Check sheet for the modelled part. Datum: model origin and axes. Units: mm. Face numbers are marked on the shaded views. A direction names the side the tool comes from. Round coordinates to 2 decimals unless told otherwise and drop trailing zeros. Write each loop counter-clockwise with the first axis right and the second up, starting at its lowest first coordinate (ties: lowest second). Pieces come first, ordered by that corner, then holes. Notation, with made-up numbers: M 29,16 L 49,16 A20 cw 49,33 Z; hole C 58.25,42 d3. An arc over 180 degrees is marked long. Answer in a Markdown table with one row per item.
```python
from build123d import *

# Parameters (mm, degrees)
F0_W     = 60
F0_H     = 30
F1_DEPTH = 30
F2_T     = -1.5
F3_R     = 6
F4_DEPTH = 1.501
F5_R     = 4
F6_DEPTH = 30.001
F7_R     = 2
F8_SIZE  = 1


with BuildPart() as f1:
    # F0 (on Top) → F1 (new body)
    with BuildSketch(Plane.XY):
        Rectangle(F0_W, F0_H)
    extrude(amount=F1_DEPTH)

    # F2
    f2_openings = [f1.faces().sort_by_distance(p)[0] for p in [
        (0, 0, 0),
    ]]
    offset(amount=F2_T, openings=f2_openings)

    # F3 (on face) → F4 (cut, through all)
    with BuildSketch(Plane(origin=(0, -13.5, 0), x_dir=(-1, 0, 0), z_dir=(0, 1, 0))):
        with Locations((-18.5, 19.5)):
            Circle(F3_R)
        with Locations((18.5, 19.5)):
            Circle(F3_R)
    extrude(amount=-F4_DEPTH, mode=Mode.SUBTRACT)

    # F5 (on face) → F6 (cut, through all)
    with BuildSketch(Plane.XY.offset(30)):
        with Locations((0, 6)):
            Circle(F5_R)
    extrude(amount=-F6_DEPTH, mode=Mode.SUBTRACT)

    # F7
    f7_edges = [f1.edges().sort_by_distance(p)[0] for p in [
        (30, 15, 15),
        (30, -15, 15),
        (-30, -15, 15),
        (-30, 15, 15),
    ]]
    fillet(f7_edges, radius=F7_R)

    # F8
    f8_edges = [f1.edges().sort_by_distance(p)[0] for p in [
        (28.5, 0, 28.5),
        (0, 13.5, 28.5),
        (0, -13.5, 28.5),
        (-28.5, 0, 28.5),
        (28.5, -13.5, 14.25),
        (28.5, 13.5, 14.25),
        (-28.5, -13.5, 14.25),
        (-28.5, 13.5, 14.25),
        (0, 15, 30),
        (30, 0, 30),
        (-30, 0, 30),
        (0, -15, 30),
    ]]
    chamfer(f8_edges, length=F8_SIZE)


solid = f1.part
```
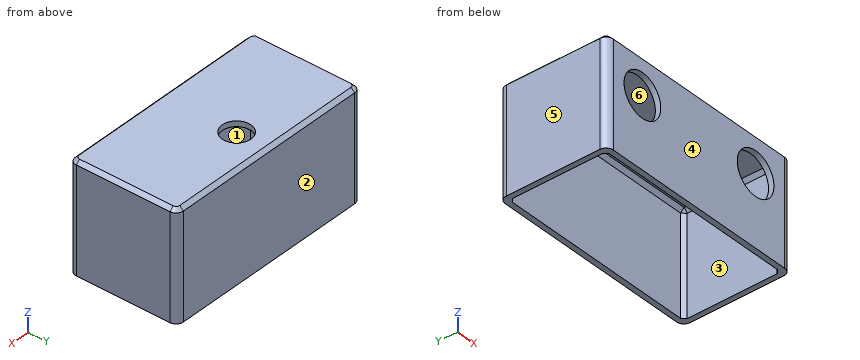
1. Draft check along X on the marked faces 3, 4, 5 and 6. Enter one of: +X half, -X half, draft (parallel to the pull), parting line (faces both ways), or undercut.
Found:
| item | result |
|---|---|
| face 3 | undercut |
| face 4 | draft |
| face 5 | -X half |
| face 6 | undercut |
2. Scan lines: L1, parallel to X at y = -7.75, z = 16.25; L2, parallel to Y at x = -5.5, z = 20.25; L3, parallel to Y at x = -20, z = 17. Record each from-to range of solid material in increasing order.
Found:
| item | result |
|---|---|
| L1 | x = -30 to -28.5, 28.5 to 30 |
| L2 | y = -15 to -13.5, 13.5 to 15 |
| L3 | y = 13.5 to 15 |
3. Section check A-A, the plane y = 6. Record the cut outline in (x, z), and give its area (4 significant figures).
Found:
| item | result |
|---|---|
| outline | M -30,0 L -28.5,0 L -28.5,27.5 L -27.5,28.5 L -4,28.5 L -4,30 L -29,30 L -30,29 Z; M 4,28.5 L 27.5,28.5 L 28.5,27.5 L 28.5,0 L 30,0 L 30,29 L 29,30 L 4,30 Z |
| area | 163.5 mm2 |
4. Section check C-C, the plane x = -18.5. Record the cut outline in (y, z), and give its area (4 significant figures).
Found:
| item | result |
|---|---|
| outline | M -15,0 L -13.5,0 L -13.5,13.5 L -15,13.5 Z; M -15,25.5 L -13.5,25.5 L -13.5,27.5 L -12.5,28.5 L 12.5,28.5 L 13.5,27.5 L 13.5,0 L 15,0 L 15,29 L 14,30 L -14,30 L -15,29 Z |
| area | 112.5 mm2 |
5. Section check D-D, the plane x = -6. Record the cut outline in (y, z), and give its area (4 significant figures).
Found:
| item | result |
|---|---|
| outline | M -15,0 L -13.5,0 L -13.5,27.5 L -12.5,28.5 L 12.5,28.5 L 13.5,27.5 L 13.5,0 L 15,0 L 15,29 L 14,30 L -14,30 L -15,29 Z |
| area | 130.5 mm2 |
6. Go/stop test with flat-tipped pins: pin 1 (8 mm diameter, centred on x = 0, y = -4, fed in from -Z); pin 2 (7 mm diameter, centred on x = 18.5, z = 19.5, fed in from -Y). Record where each tip stops, or that it passes through.
Found:
| item | result |
|---|---|
| pin 1 | stops at z = 28.5 |
| pin 2 | stops at y = 13.5 |
7. Access from +Z, -Z, +X, -X, +Y, -Y to the whole of each face (thin tool, end or side, straight path). Record for the marked faces 1 and 2.
Found:
| item | result |
|---|---|
| face 1 | -Z |
| face 2 | +Z, -Z, +X, -X, +Y |
8. Section check B-B, the plane z = 12.25. Record the cut outline in (x, y), and give its area (3 significant figures).
Found:
| item | result |
|---|---|
| outline | M -30,-13 A2 ccw -28,-15 L 28,-15 A2 ccw 30,-13 L 30,13 A2 ccw 28,15 L -28,15 A2 ccw -30,13 Z; hole M -28.5,-12.5 L -27.5,-13.5 L 27.5,-13.5 L 28.5,-12.5 L 28.5,12.5 L 27.5,13.5 L -27.5,13.5 L -28.5,12.5 Z |
| area | 260 mm2 |
